from build123d import *

# Parameters (mm, degrees)
SKETCH1_W           = 26
SKETCH1_H           = 16.09
BOSS_EXTRUDE1_DEPTH = 46
SKETCH2_R           = 5.5
BOSS_EXTRUDE2_DEPTH = 2


with BuildPart() as part:
    # Sketch1 → Boss-Extrude1 (new body)
    with BuildSketch(Plane.XY):
        Rectangle(SKETCH1_W, SKETCH1_H)
    extrude(amount=BOSS_EXTRUDE1_DEPTH)

    # Sketch2 → Boss-Extrude2 (add)
    with BuildSketch(Plane.XY.offset(46)):
        with Locations((6.529444473, 0)):
            Circle(SKETCH2_R)
        Polygon((-7.134758176, -5.773481444), (-2.126944774, -2.900305802), (-2.111281169, 2.873175642), (-7.103430965, 5.773481444), (-12.111244367, 2.900305802), (-12.126907972, -2.873175642), align=None)
    extrude(amount=BOSS_EXTRUDE2_DEPTH)


solid = part.part
For this review, take the finished solid that the model builds, in its own axes (mm). A direction names the side the tool comes from. Give positions to 0.01 mm unless a question says otherwise; leave off trailing zeros. Order: outer loops, then holes, each group sorted by start corner. A loop starts at its lowest first (then second) coordinate and runs counter-clockwise, first axis right, second up. Notation, with made-up numbers: (49.5, -30.75) - (55.5, -30.75) arc R23 cw to (55.5, -14.75) - close; hole circle Ø6 at (9.25, 43.5). An arc over 180 degrees is marked (long way). Answer as a JSON object with one key per item and string values. Group by question number.
Item 1: Take a section at B-B on y = 6.75. Give the boundary of the cut face in (x, z), and give its area (3 significant figures).
Item 2: Clearance check with a flat-ended pin moving along its axis: pin 1 Ø8 at (x, y) = (-2.5, -3) entering from -Z. State where the tip first meets the part, or that it passes through.
Item 3: Machinability: for faces 1 (the flat face through (-4.67, -4.36, 46.99)), 2 (the flat face through (-9.67, -4.3, 46.99)), 3 (the flat face through (-4.57, 4.3, 46.99)), 4 (the flat face through (-9.57, 4.36, 46.99)), 5 (the cylindrical face through (1.035, 0.242, 46.986)), which of the approach directions +Z, -Z, +X, -X, +Y, -Y give a long, thin tool a straight path to every point of the face, cutting with its end or side? Answer none if there is none.
Item 4: Take a section at A-A on x = -10.5. Give the boundary of the cut face in (y, z) (3 decimals), and give its area (3 significant figures).
Item 5: Take a section at C-C on x = 8.5. Give the boundary of the cut face in (y, z) (3 decimals), and give its area (3 significant figures).
Item 6: Draft analysis for pull direction X (two halves, no side actions). For faces 6 (the flat face through (-7, 0, 48)), 7 (the flat face through (-13, 0, 23)), 8 (the flat face through (0, 0, 46)), state which applies: pulls with the +X half, pulls with the -X half, needs draft (parallel to the pull), parting line crosses it, or undercut.
Item 7: Wall thickness on line 1 along Z through (x, y) = (-0.5, -5.75): over which ranges is the line inside the solid? List them lowest first.
Reported:
{
 "1": {"outline": "(-13, 0) - (13, 0) - (13, 46) - (-13, 46) - close", "area": "1,200 mm^2"},
 "2": {"pin 1": "z = 0"},
 "3": {"face 1": "+Z, -Y", "face 2": "+Z, -X, -Y", "face 3": "+Z, +Y", "face 4": "+Z, -X, +Y", "face 5": "+Z"},
 "4": {"outline": "(-8.045, 0) - (8.045, 0) - (8.045, 46) - (3.825, 46) - (3.825, 48) - (-3.818, 48) - (-3.818, 46) - (-8.045, 46) - close", "area": "755 mm^2"},
 "5": {"outline": "(-8.045, 0) - (8.045, 0) - (8.045, 46) - (5.135, 46) - (5.135, 48) - (-5.135, 48) - (-5.135, 46) - (-8.045, 46) - close", "area": "761 mm^2"},
 "6": {"face 6": "needs draft", "face 7": "pulls with the -X half", "face 8": "undercut"},
 "7": {"line 1": "0 to 46"}
}
